Autodesk Inventor part; units mm, degrees
ref_plane "YZ Plane" through (0, 0, 0) normal (1, 0, 0) x (0, 1, 0)
ref_plane "XZ Plane" through (0, 0, 0) normal (0, 1, 0) x (-1, 0, 0)
ref_plane "XY Plane" through (0, 0, 0) normal (0, 0, 1) x (1, 0, 0)
sketch "スケッチ1" plane through (0, 0, 0) normal (0, 0, 1) x (1, 0, 0)
  line L0 (-56.5, -17) -> (56.5, -17)
  line L1 (56.5, -17) -> (56.5, 17)
  line L2 (56.5, 17) -> (-56.5, 17)
  line L3 (-56.5, 17) -> (-56.5, -17)
  line L4 (-56.5, -17) -> (56.5, 17) construction
  line L5 (56.5, -17) -> (-56.5, 17) construction
  point P0 (0, 0)
  dimension "d0" = 113
  dimension "d1" = 34
extrude "押し出し1" add sketch "スケッチ1" along normal blind 14
mirror "ミラー1" about plane through (0, 0, 0) normal (0, 0, -1) of "押し出し1"
fillet "フィレット1" radius 14 2 edges at (-56.5, 0, 14) (-56.5, 0, -14)
fillet "フィレット2" radius 2 2 edges at (56.5, 0, 14) (56.5, 0, -14)
properties part number "バッテリー(G6 HI-VOLTAGE 2400MAH 3S 80CMAX LIPO)"
Geometry: final body of the model. Coordinates: model frame, mm. Give positions to 0.01 mm unless a question says otherwise; leave off trailing zeros. Write each loop counter-clockwise with the first axis right and the second up, starting at its lowest first coordinate (ties: lowest second). Pieces come first, ordered by that corner, then holes. Notation, with made-up numbers: M 45.5,87 L 57.5,87 A31 cw 57.5,112 Z; hole C -3,76.5 d1. An arc over 180 degrees is marked long. Answer in a Markdown table with one row per item. Add a question column.
(1) Section B-B on z = 9.75. Return loops of the section in (x, y).
(2) First-contact query: pin 1 (3 mm diameter, centred on y = 6.5, z = 8, fed in from -X). Flat tip, straight axial feed; report the tip coordinate or a pass-through.
(3) Ray query, line 1 (X direction, y = 5, z = 9.25); line 2 (X direction, y = -10, z = -5.75). Return the intervals inside material, ascending.
(4) Section C-C on x = -47. Return loops of the section in (y, z).
Result set:
| question | item | result |
|---|---|---|
| 1 | outline | M -52.55,-17 L 56.5,-17 L 56.5,17 L -52.55,17 Z |
| 2 | pin 1 | stops at x = -54.9 |
| 3 | line 1 | x = -53.01 to 56.5 |
| 3 | line 2 | x = -55.26 to 56.5 |
| 4 | outline | M -17,-13.26 L 17,-13.26 L 17,13.26 L -17,13.26 Z |
